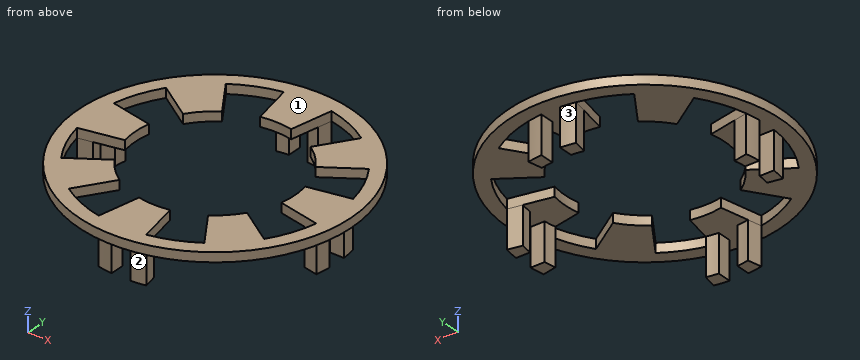
from build123d import *

# Parameters (mm, degrees)
SKETCH1_R           = 14.5
BOSS_EXTRUDE1_DEPTH = 1
BOSS_EXTRUDE2_START = 4
BOSS_EXTRUDE2_DEPTH = 4


with BuildPart() as part:
    # Sketch1 → Boss-Extrude1 (new body)
    with BuildSketch(Plane.XY):
        Circle(SKETCH1_R)
        with BuildLine():
            ThreePointArc((-1.658267737, 8.336674883), (0, 8.5), (1.658267737, 8.336674883))
            Line((1.658267737, 8.336674883), (2.536174186, 12.750208645))
            ThreePointArc((2.536174186, 12.750208645), (4.974884621, 12.010433923), (7.222413029, 10.80910496))
            Line((7.222413029, 10.80910496), (4.722346981, 7.067491705))
            ThreePointArc((4.722346981, 7.067491705), (6.01040764, 6.01040764), (7.067491705, 4.722346981))
            Line((7.067491705, 4.722346981), (10.80910496, 7.222413029))
            ThreePointArc((10.80910496, 7.222413029), (12.010433923, 4.974884621), (12.750208645, 2.536174186))
            Line((12.750208645, 2.536174186), (8.336674883, 1.658267737))
            ThreePointArc((8.336674883, 1.658267737), (8.5, 0), (8.336674883, -1.658267737))
            Line((8.336674883, -1.658267737), (12.750208645, -2.536174186))
            ThreePointArc((12.750208645, -2.536174186), (12.010433923, -4.974884621), (10.80910496, -7.222413029))
            Line((10.80910496, -7.222413029), (7.067491705, -4.722346981))
            ThreePointArc((7.067491705, -4.722346981), (6.01040764, -6.01040764), (4.722346981, -7.067491705))
            Line((4.722346981, -7.067491705), (7.222413029, -10.80910496))
            ThreePointArc((7.222413029, -10.80910496), (4.974884621, -12.010433923), (2.536174186, -12.750208645))
            Line((2.536174186, -12.750208645), (1.658267737, -8.336674883))
            ThreePointArc((1.658267737, -8.336674883), (0, -8.5), (-1.658267737, -8.336674883))
            Line((-1.658267737, -8.336674883), (-2.536174186, -12.750208645))
            ThreePointArc((-2.536174186, -12.750208645), (-4.974884621, -12.010433923), (-7.222413029, -10.80910496))
            Line((-7.222413029, -10.80910496), (-4.722346981, -7.067491705))
            ThreePointArc((-4.722346981, -7.067491705), (-6.01040764, -6.01040764), (-7.067491705, -4.722346981))
            Line((-7.067491705, -4.722346981), (-10.80910496, -7.222413029))
            ThreePointArc((-10.80910496, -7.222413029), (-12.010433923, -4.974884621), (-12.750208645, -2.536174186))
            Line((-12.750208645, -2.536174186), (-8.336674883, -1.658267737))
            ThreePointArc((-8.336674883, -1.658267737), (-8.5, 0), (-8.336674883, 1.658267737))
            Line((-8.336674883, 1.658267737), (-12.750208645, 2.536174186))
            ThreePointArc((-12.750208645, 2.536174186), (-12.010433923, 4.974884621), (-10.80910496, 7.222413029))
            Line((-10.80910496, 7.222413029), (-7.067491705, 4.722346981))
            ThreePointArc((-7.067491705, 4.722346981), (-6.01040764, 6.01040764), (-4.722346981, 7.067491705))
            Line((-4.722346981, 7.067491705), (-7.222413029, 10.80910496))
            ThreePointArc((-7.222413029, 10.80910496), (-4.974884621, 12.010433923), (-2.536174186, 12.750208645))
            Line((-2.536174186, 12.750208645), (-1.658267737, 8.336674883))
        make_face(mode=Mode.SUBTRACT)
    extrude(amount=BOSS_EXTRUDE1_DEPTH)

    # Sketch2 → Boss-Extrude2 (add)
    with BuildSketch(Plane(origin=(0, 0, 0), x_dir=(-1, 0, 0), z_dir=(0, 0, -1)).offset(BOSS_EXTRUDE2_START)):
        with BuildLine():
            Line((2.536174186, -12.750208645), (2.243538703, -11.279030725))
            ThreePointArc((2.243538703, -11.279030725), (1.624193423, -11.384726423), (1, -11.456439237))
            Line((1, -11.456439237), (1, -12.961481397))
            ThreePointArc((1, -12.961481397), (1.771239965, -12.8787697), (2.536174186, -12.750208645))
        make_face()
        with BuildLine():
            Line((-1, -12.961481397), (-1, -11.456439237))
            ThreePointArc((-1, -11.456439237), (-1.624193423, -11.384726423), (-2.243538703, -11.279030725))
            Line((-2.243538703, -11.279030725), (-2.536174186, -12.750208645))
            ThreePointArc((-2.536174186, -12.750208645), (-1.771239965, -12.8787697), (-1, -12.961481397))
        make_face()
        with BuildLine():
            Line((12.961481397, -1), (11.456439237, -1))
            ThreePointArc((11.456439237, -1), (11.384726423, -1.624193423), (11.279030725, -2.243538703))
            Line((11.279030725, -2.243538703), (12.750208645, -2.536174186))
            ThreePointArc((12.750208645, -2.536174186), (12.8787697, -1.771239965), (12.961481397, -1))
        make_face()
        with BuildLine():
            Line((12.750208645, 2.536174186), (11.279030725, 2.243538703))
            ThreePointArc((11.279030725, 2.243538703), (11.384726423, 1.624193423), (11.456439237, 1))
            Line((11.456439237, 1), (12.961481397, 1))
            ThreePointArc((12.961481397, 1), (12.8787697, 1.771239965), (12.750208645, 2.536174186))
        make_face()
        with BuildLine():
            ThreePointArc((1, 11.456439237), (1.624193423, 11.384726423), (2.243538703, 11.279030725))
            Line((2.243538703, 11.279030725), (2.536174186, 12.750208645))
            ThreePointArc((2.536174186, 12.750208645), (1.771239965, 12.8787697), (1, 12.961481397))
            Line((1, 12.961481397), (1, 11.456439237))
        make_face()
        with BuildLine():
            ThreePointArc((-2.243538703, 11.279030725), (-1.624193423, 11.384726423), (-1, 11.456439237))
            Line((-1, 11.456439237), (-1, 12.961481397))
            ThreePointArc((-1, 12.961481397), (-1.771239965, 12.8787697), (-2.536174186, 12.750208645))
            Line((-2.536174186, 12.750208645), (-2.243538703, 11.279030725))
        make_face()
        with BuildLine():
            ThreePointArc((-11.456439237, 1), (-11.384726423, 1.624193423), (-11.279030725, 2.243538703))
            Line((-11.279030725, 2.243538703), (-12.750208645, 2.536174186))
            ThreePointArc((-12.750208645, 2.536174186), (-12.8787697, 1.771239965), (-12.961481397, 1))
            Line((-12.961481397, 1), (-11.456439237, 1))
        make_face()
        with BuildLine():
            ThreePointArc((-11.279030725, -2.243538703), (-11.384726423, -1.624193423), (-11.456439237, -1))
            Line((-11.456439237, -1), (-12.961481397, -1))
            ThreePointArc((-12.961481397, -1), (-12.8787697, -1.771239965), (-12.750208645, -2.536174186))
            Line((-12.750208645, -2.536174186), (-11.279030725, -2.243538703))
        make_face()
    extrude(amount=-BOSS_EXTRUDE2_DEPTH)


solid = part.part
Source: CAD feature listing. Evaluate the final solid. Frame: model axes, mm. Face numbers are marked on the shaded views. A direction names the side the tool comes from. Coordinates: 2 decimals unless noted, no trailing zeros. Loops run counter-clockwise (first coordinate to the right, second up) from the corner with the lowest first, then second, coordinate; pieces in that order, holes last. Notation, with made-up numbers: (-25, -8) -> (-6, -8) arc R13 ccw to (-6, 8) -> close; hole circle Ø11 at (9, 89). An arc over 180 degrees is marked (long way). Answer in a Markdown table with one row per item. Add a question column.
Q1. Section D-D on x = 6. Return the cut outline in (y, z), and give its area (3 significant figures).
Q2. Ray query, line 1 along Z through (x, y) = (12, 0.5); line 2 along Y through (x, z) = (-1.5, -0.8); line 3 along X through (y, z) = (7, 0.7). Return the intervals inside material, ascending.
Q3. Section B-B on z = -3.05. Give the number of separate pieces and of enclosed holes in the cut face, and give its area (4 significant figures).
Q4. Reachability of the marked faces 1, 2 and 3 from +Z, -Z, +X, -X, +Y, -Y: full face, straight path, thin tool, end or side. Return the list, or none.
Q5. Section A-A on y = 0. Return the cut outline in (x, z), and give its area (3 significant figures).
Q6. Contact query for flat-ended pins moving along their axis: pin 1 Ø0.8 at (x, z) = (12.5, -1.5) entering from -Y; pin 2 Ø1.2 at (y, z) = (-12.5, -3) entering from +X; pin 3 Ø0.5 at (y, z) = (12, -3) entering from -X; pin 4 Ø1.5 at (x, z) = (-10, -3) entering from +Y. Output: stop coordinate, or through.
Computed values:
| question | item | result |
|---|---|---|
| 1 | outline | (-13.2, 0) -> (-11.53, 0) -> (-11.53, 1) -> (-13.2, 1) -> close; (-8.98, 0) -> (-6.02, 0) -> (-6.02, 1) -> (-8.98, 1) -> close; (6.02, 0) -> (8.98, 0) -> (8.98, 1) -> (6.02, 1) -> close; (11.53, 0) -> (13.2, 0) -> (13.2, 1) -> (11.53, 1) -> close |
| 1 | area | 9.25 mm^2 |
| 2 | line 1 | z = 0 to 1 |
| 2 | line 2 | y = -12.91 to -11.4, 11.4 to 12.91 |
| 2 | line 3 | x = -12.7 to -10.95, -10.48 to -4.82, 4.82 to 10.48, 10.95 to 12.7 |
| 3 | separate pieces | 8 |
| 3 | enclosed holes | 0 |
| 3 | area | 16.85 mm^2 |
| 4 | face 1 | +Z, +X, -X, +Y, -Y |
| 4 | face 2 | -Z, +X, -Y |
| 4 | face 3 | -Z, -X, +Y |
| 5 | outline | (-14.5, 0) -> (-8.5, 0) -> (-8.5, 1) -> (-14.5, 1) -> close; (8.5, 0) -> (14.5, 0) -> (14.5, 1) -> (8.5, 1) -> close |
| 5 | area | 12.0 mm^2 |
| 6 | pin 1 | stops at y = -2.54 |
| 6 | pin 2 | stops at x = 2.54 |
| 6 | pin 3 | stops at x = -2.44 |
| 6 | pin 4 | passes through |
